Can you work these out from the model? Positions are in its coordinate system, mm. A direction names the side the tool comes from. Coordinates: 2 decimals unless noted, no trailing zeros. Order: outer loops, then holes, each group sorted by start corner. A loop starts at its lowest first (then second) coordinate and runs counter-clockwise, first axis right, second up. Notation, with made-up numbers: (32.25, 42) -> (84.25, 42) arc R21 cw to (84.25, 68) -> close; hole circle Ø1 at (77.25, 21). An arc over 180 degrees is marked (long way). Answer in a Markdown table with one row per item. Add a question column.
1. We'd pull the mould along Y, two halves only. Please class faces 1 (the face through (-54.94, -1, 1)), 2 (the face through (52.5, -30, -89)), 3 (the face through (101.928, 48.365, -63.077)): pulls with the +Y half, pulls with the -Y half, needs draft (parallel to the pull), parting line crosses it, or undercut.
2. Imagine slicing it at A-A on x = -6.5. Write out the boundary of the cut face in (y, z), plus the area to 3 significant figures.
3. Will these pins go through, and if not, where does the flat tip stop? pin 1 (12.5 mm diameter, centred on x = 4, z = 106.5, fed in from +Y); pin 2 (1.5 mm diameter, centred on x = -65, z = 57, fed in from -Y); pin 3 (6 mm diameter, centred on x = 110, z = 12, fed in from +Y).
4. On a 3-axis mill with a long thin cutter (end or side, diameter ignored), from which of +Z, -Z, +X, -X, +Y, -Y can I reach the whole of each face in a straight line? I mean faces 4 (the face through (-105.64, -71.56, -9.4)), 5 (the face through (-52.5, -30, -90)), 6 (the face through (110.531, 76.908, -17.078)). Say none if no direction works.
5. If I drill on line 1 along Y through (x, z) = (-110, 0); line 2 along X through (y, z) = (22, 52.5), over which ranges is the centre line in solid material (lowest first)? Write a range as [from, to].
6. Imagine slicing it at B-B on x = 136.5. Write out the boundary of the cut face in (y, z), plus the area to 3 significant figures.
from build123d import *

# Parameters (mm, degrees)
PAD_DEPTH = 41.402


with BuildPart() as part:
    # Sketch → Revolution (revolve)
    with BuildSketch(Plane.XZ):
        Polygon((-103.94, 78.781697), (-62.5, 93.264797), (-62.5, 99.568), (-52.5, 99.568), (-52.5, 93.264797), (52.5, 93.264797), (52.5, 99.568), (62.5, 99.568), (62.5, 93.264797), (103.94, 78.781697), (116.94, 78.781697), (122.94, 74.676), (154.94, 74.676), (154.94, 72.176), (54.94, 72.176), (54.94, 0), (-54.94, 0), (-54.94, 72.176), (-154.94, 72.176), (-154.94, 74.676), (-122.94, 74.676), (-116.94, 78.781697), align=None)
    revolve(axis=Axis((0, 0, 0), (1, 0, 0)))

    # Sketch001 → Pad (new body)
    with BuildSketch(Plane.XY.offset(76.2)):
        with BuildLine():
            Line((-50.3, -59.944), (50.3, -59.944))
            ThreePointArc((50.3, -59.944), (59.280256, -56.224256), (63, -47.244))
            Line((63, -47.244), (63, 47.244))
            ThreePointArc((63, 47.244), (59.280256, 56.224256), (50.3, 59.944))
            Line((50.3, 59.944), (-50.3, 59.944))
            ThreePointArc((-50.3, 59.944), (-59.280256, 56.224256), (-63, 47.244))
            Line((-63, 47.244), (-63, -47.244))
            ThreePointArc((-63, -47.244), (-59.280256, -56.224256), (-50.3, -59.944))
        make_face()
    extrude(amount=PAD_DEPTH)


solid = part.part
Answers follow:
| question | item | result |
|---|---|---|
| 1 | face 1 | undercut |
| 1 | face 2 | needs draft |
| 1 | face 3 | parting line crosses it |
| 2 | outline | (-59.94, 76.2) -> (-53.78, 76.2) arc R93.26 ccw (long way) to (53.78, 76.2) -> (59.94, 76.2) -> (59.94, 117.6) -> (-59.94, 117.6) -> close |
| 2 | area | 31,000 mm² |
| 3 | pin 1 | stops at y = 59.94 |
| 3 | pin 2 | stops at y = -73.38 |
| 3 | pin 3 | stops at y = 78.27 |
| 4 | face 4 | -X |
| 4 | face 5 | none |
| 4 | face 6 | +X |
| 5 | line 1 | y = [-78.78, -72.18], [72.18, 78.78] |
| 5 | line 2 | x = [-54.94, 54.94] |
| 6 | outline | circle Ø149.35 at (0, 0); hole circle Ø144.35 at (0, 0) |
| 6 | area | 1,150 mm² |
